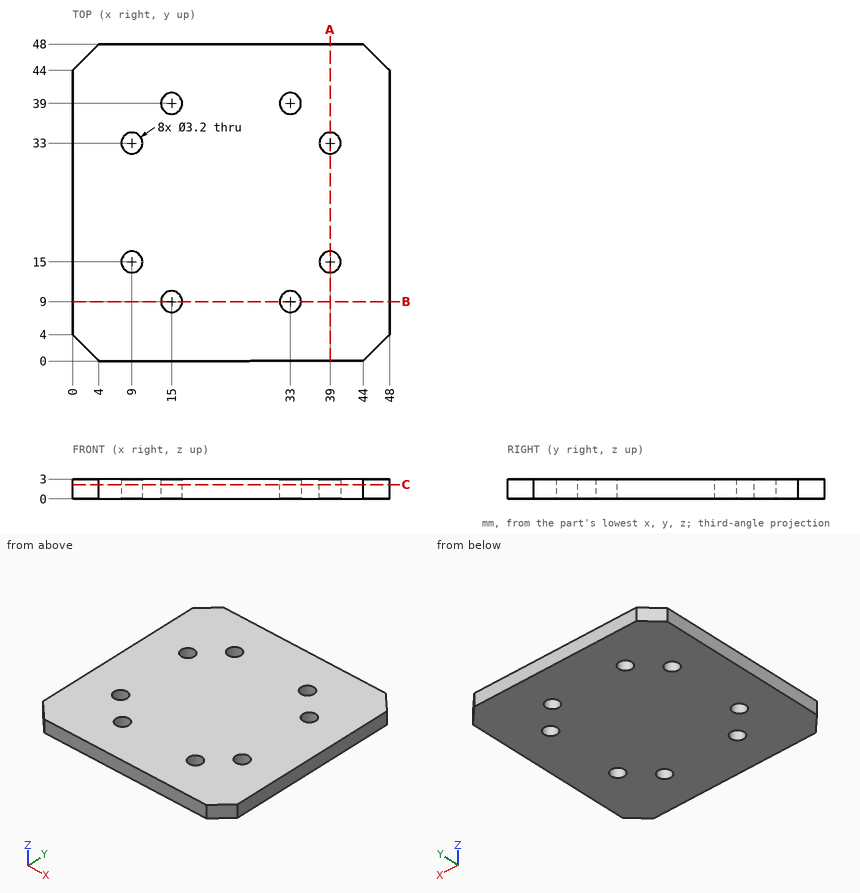
Here's the drawing with two shaded views (mm, measured from the low corner). I have some questions. Round coordinates to 2 decimals unless told otherwise and drop trailing zeros. Loops run counter-clockwise (first coordinate to the right, second up) from the corner with the lowest first, then second, coordinate; pieces in that order, holes last. Notation, with made-up numbers: M -27,-36 L 5,-36 A25 cw 5,-9 Z; hole C 83,47 d5. An arc over 180 degrees is marked long. Put each result on its own line as item: value.
Q1. Imagine slicing it at A-A (x = 39). Write out the boundary of the cut face in (y, z).
Check result:
outline: M 0,0 L 13.4,0 L 13.4,3 L 0,3 Z; M 16.6,0 L 31.4,0 L 31.4,3 L 16.6,3 Z; M 34.6,0 L 48,0 L 48,3 L 34.6,3 Z
Q2. Imagine slicing it at C-C (z = 2.15). State how many separate pieces and enclosed holes the cut face has, then the cut area to 3 significant figures.
Check result:
separate pieces: 1
enclosed holes: 8
area: 2,210 mm2
Q3. For pin 1 (3 mm diameter, centred on x = 33, y = 9, fed in from -Z); pin 2 (4 mm diameter, centred on x = 39, y = 15, fed in from -Z), each with a flat end and sliding along its axis, tell me the tip position at first contact or that it passes through.
Check result:
pin 1: through
pin 2: z = 0
Q4. I need wall thicknesses on probe 1 along X at (y, z) = (33, 1.6); probe 2 along X at (y, z) = (14, 0.6). Which ranges of each line are inside material? Lowest first, please.
Check result:
probe 1: 0 to 7.4, 10.6 to 37.4, 40.6 to 48
probe 2: 0 to 7.75, 10.25 to 37.75, 40.25 to 48
